The model under review builds one solid part; all positions refer to its coordinate system, in mm. Face numbers are marked on the shaded views. Round coordinates to 2 decimals unless told otherwise and drop trailing zeros. Loops run counter-clockwise (first coordinate to the right, second up) from the corner with the lowest first, then second, coordinate; pieces in that order, holes last. Notation, with made-up numbers: (79, -27) -> (97, -27) arc R37 cw to (97, 10) -> close; hole circle Ø2 at (83.5, 22.5). An arc over 180 degrees is marked (long way). Use a Markdown table: item, result. Add a question column.
1) Consider section D-D on z = 24.5. Give the boundary of the cut face in (x, y).
2) Mouldability with a two-part tool opening along X and no side actions: class the marked faces 1, 2 and 3 as released by +X, released by -X, zero draft, split by the parting line, or undercut.
3) Wall thickness on probe 1 along Z at (x, y) = (29, -27); probe 2 along Z at (x, y) = (4.5, -34); probe 3 along Y at (x, z) = (0, 32): over which ranges is each line inside the solid? List them lowest first.
4) Consider section A-A on x = 0. Give the boundary of the cut face in (y, z).
5) Insertion check: pin 1 (4 mm diameter, centred on y = 8, z = 23, fed in from +X); pin 2 (12 mm diameter, centred on y = 20.5, z = 35, fed in from +X); pin 3 (3 mm diameter, centred on x = 19.5, y = -25, fed in from -Z); pin 4 (3 mm diameter, centred on y = 5.5, z = 32.5, fed in from -X). Each pin has a flat end and moves straight along its axis. Give the tip position at first contact, or say it passes through.
6) Consider section C-C on z = 34.5. Give the boundary of the cut face in (x, y), plus the area to 3 significant figures.
from build123d import *

# Parameters (mm, degrees)
SKETCH1_R           = 40
SKETCH1_R_2         = 10
BOSS_EXTRUDE1_DEPTH = 40
SKETCH2_R           = 10


with BuildPart() as part:
    # Sketch1 → Boss-Extrude1 (new body)
    with BuildSketch(Plane.XY):
        Circle(SKETCH1_R)
        Circle(SKETCH1_R_2, mode=Mode.SUBTRACT)
    extrude(amount=BOSS_EXTRUDE1_DEPTH)

    # Sketch2 → Cut-Revolve1 (revolve, cut)
    with BuildSketch(Plane(origin=(0, 0, 0), x_dir=(1, 0, 0), z_dir=(0, 1, 0))):
        with Locations((-40, -20)):
            Circle(SKETCH2_R)
    revolve(axis=Axis((0, 0, 0), (0, 0, 1)), mode=Mode.SUBTRACT)


solid = part.part
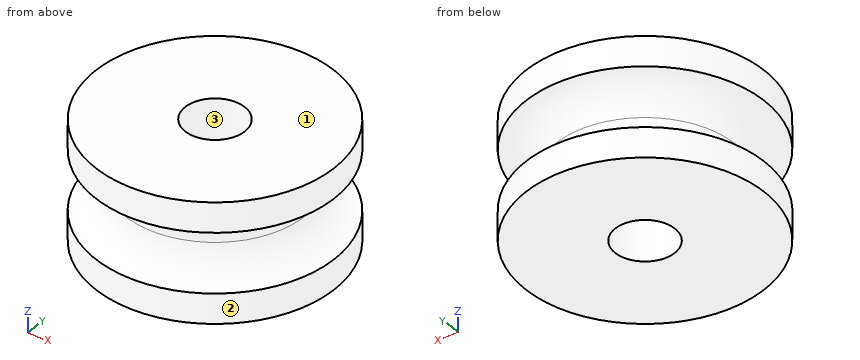
Result set:
| question | item | result |
|---|---|---|
| 1 | outline | circle Ø62.14 at (0, 0); hole circle Ø20 at (0, 0) |
| 2 | face 1 | zero draft |
| 2 | face 2 | split by the parting line |
| 2 | face 3 | undercut |
| 3 | probe 1 | 0 to 10.01, 29.99 to 40 |
| 3 | probe 2 | 0 to 11.79, 28.21 to 40 |
| 3 | probe 3 | -40 to -10, 10 to 40 |
| 4 | outline | (-40, 0) -> (-10, 0) -> (-10, 40) -> (-40, 40) -> (-40, 30) arc R10 cw to (-40, 10) -> close; (10, 0) -> (40, 0) -> (40, 10) arc R10 cw to (40, 30) -> (40, 40) -> (10, 40) -> close |
| 5 | pin 1 | x = 30.4 |
| 5 | pin 2 | x = 37.28 |
| 5 | pin 3 | z = 0 |
| 5 | pin 4 | x = -39.8 |
| 6 | outline | circle Ø80 at (0, 0); hole circle Ø20 at (0, 0) |
| 6 | area | 4,710 mm2 |
